Input: part model. Units: mm. Frame: model coordinates. Round coordinates to 2 decimals unless told otherwise and drop trailing zeros. Loops run counter-clockwise (first coordinate to the right, second up) from the corner with the lowest first, then second, coordinate; pieces in that order, holes last.
1) First-contact query: pin 1 (8 mm diameter, centred on x = 50.8, z = 0, fed in from +Y); pin 2 (1 mm diameter, centred on y = 1.5, z = -1, fed in from +X); pin 3 (0.8 mm diameter, centred on x = -2.5, y = 1, fed in from -Z). Flat tips, straight axial feed; report the tip coordinate or a pass-through.
2) Section D-D, the plane x = 50.8. Return loops of the section in (y, z), and give its area (3 significant figures).
3) Ray query, line 1 along Z through (x, y) = (50.8, 1.5); line 2 along Z through (x, y) = (-50.5, 0.7); line 3 along X through (y, z) = (0.2, 2). Return the intervals inside material, ascending.
4) Section C-C, the plane y = 2.05. Return loops of the section in (x, z).
5) Section A-A, the plane x = -50.8. Return loops of the section in (y, z), and give its area (3 significant figures).
6) Section B-B, the plane z = 0. Return loops of the section in (x, y).
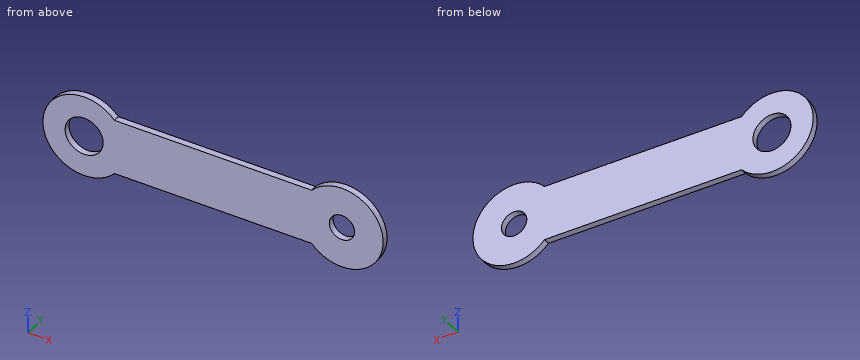
from build123d import *

# Parameters (mm, degrees)
BOSS_EXTRUDE1_DEPTH = 2.54
SKETCH2_R           = 7.5
SKETCH2_R_2         = 5
CUT_EXTRUDE1_DEPTH  = 2.54


with BuildPart() as part:
    # Sketch1 → Boss-Extrude1 (new body)
    with BuildSketch(Plane(origin=(0, 0, 0), x_dir=(1, 0, 0), z_dir=(0, 1, 0))):
        with BuildLine():
            Line((-38.836017724, 11), (38.836017598, 11))
            ThreePointArc((38.836017598, 11), (67.052288298, 0), (38.836017598, -11))
            Line((38.836017598, -11), (-38.836017724, -11))
            ThreePointArc((-38.836017724, -11), (-67.052288205, 0), (-38.836017724, 11))
        make_face()
    extrude(amount=BOSS_EXTRUDE1_DEPTH)

    # Sketch2 → Cut-Extrude1 (cut)
    with BuildSketch(Plane(origin=(0, 2.54, 0), x_dir=(1, 0, 0), z_dir=(0, 1, 0))):
        with Locations((-50.8, 0)):
            Circle(SKETCH2_R)
        with Locations((50.8, 0)):
            Circle(SKETCH2_R_2)
    extrude(amount=-CUT_EXTRUDE1_DEPTH, mode=Mode.SUBTRACT)


solid = part.part
Final values:
1. pin 1: passes through
1. pin 2: stops at x = 67.04
1. pin 3: stops at z = -11
2. outline: (0, -16.25) - (2.54, -16.25) - (2.54, -5) - (0, -5) - close; (0, 5) - (2.54, 5) - (2.54, 16.25) - (0, 16.25) - close
2. area: 57.2 mm2
3. line 1: z = -16.25 to -5, 5 to 16.25
3. line 2: z = -16.25 to -7.49, 7.49 to 16.25
3. line 3: x = -66.93 to -58.03, -43.57 to 46.22, 55.38 to 66.93
4. outline: (-38.84, -11) - (38.84, -11) arc R16.25 ccw (long way) to (38.84, 11) - (-38.84, 11) arc R16.25 ccw (long way) to start; hole circle Ø15 at (-50.8, 0); hole circle Ø10 at (50.8, 0)
5. outline: (0, -16.25) - (2.54, -16.25) - (2.54, -7.5) - (0, -7.5) - close; (0, 7.5) - (2.54, 7.5) - (2.54, 16.25) - (0, 16.25) - close
5. area: 44.5 mm2
6. outline: (-67.05, 0) - (-58.3, 0) - (-58.3, 2.54) - (-67.05, 2.54) - close; (-43.3, 0) - (45.8, 0) - (45.8, 2.54) - (-43.3, 2.54) - close; (55.8, 0) - (67.05, 0) - (67.05, 2.54) - (55.8, 2.54) - close
